Build history of the part. All positions in model axes, mm. A direction names the side the tool comes from. Coordinates: 2 decimals unless noted, no trailing zeros. Loops run counter-clockwise (first coordinate to the right, second up) from the corner with the lowest first, then second, coordinate; pieces in that order, holes last.
(1) Wall check: L1, parallel to Y at x = 0, z = 1.5; L2, parallel to Y at x = 0, z = -1. Give the ranges that are in metal, low to high.
(2) Flat gauge pins, fed straight in: P1, Ø10, axis at x = -23, z = 10, coming from the +Y side; P2, Ø18.5, axis at y = 19.5, z = 55, coming from the -X side; P3, Ø10, axis at x = 9, y = -2.5, coming from the -Z side; P4, Ø2, axis at y = 6.5, z = 42, coming from the -X side. Where does each tip first touch, or does it go through?
(3) Tool access for faces 4 (the face through (-20, -0.75, 45)), 5 (the face through (-7.14, -7, 72.57)), 6 (the face through (-9.213, -9.407, 64.333)), 7 (the face through (0.75, 20, 45)): list every direction of +Z, -Z, +X, -X, +Y, -Y with a clear straight run to the whole face (end or side of a thin tool).
(4) Slice it at A-A (z = 44). Give the cut face in (x, y), and give its area (3 significant figures).
(5) Two-plate mould, pull along Y, no slides. Class faces 1 (the face through (-8, -8, -5)), 2 (the face through (19.115, -18.713, 76.37)), 3 (the face through (-9.407, 9.213, 64.333)): pulls with the +Y half, pulls with the -Y half, needs draft (parallel to the pull), parting line crosses it, or undercut.
from build123d import *

# Parameters (mm, degrees)
AXLE_BASE_SKETCH_R        = 26
AXLE_DEPTH                = 77.5
GUARD_BASE_R              = 37.5
GUARD_DEPTH               = 5
INNER_AXLE_HOLE_BASE_R    = 10
INNER_AXLE_HOLE_DEPTH     = 83.5
BEND_START                = -64.5
BEND_ROOM_BASE_W          = 1.5
BEND_ROOM_BASE_H          = 75
BEND_ROOM_1_DEPTH         = 64.5
BEND_ROOM_2_COUNT         = 2
BEND_ROOM_2_ANGLE         = 90
EASY_REMOVAL_CHAMFER_SIZE = 4


with BuildPart() as part:
    # Axle base sketch → Axle (new body)
    with BuildSketch(Plane.XY):
        Circle(AXLE_BASE_SKETCH_R)
    extrude(amount=AXLE_DEPTH)

    # Guard base → Guard (add)
    with BuildSketch(Plane(origin=(0, 0, 0), x_dir=(-1, 0, 0), z_dir=(0, 0, -1))):
        Circle(GUARD_BASE_R)
    extrude(amount=GUARD_DEPTH)

    # Inner axle hole base → Inner axle hole (cut, through all)
    with BuildSketch(Plane.XY.offset(77.5)):
        Circle(INNER_AXLE_HOLE_BASE_R)
    extrude(amount=-INNER_AXLE_HOLE_DEPTH, mode=Mode.SUBTRACT)

    # Mate ring base → Mate rings (revolve)
    with BuildSketch(Plane(origin=(0, 0, 0), x_dir=(1, 0, 0), z_dir=(0, 1, 0))):
        Polygon((26, -77.5), (26.75, -76.75), (26.75, -76), (26, -75.25), align=None)
        Polygon((26, -71.75), (26.75, -71), (26.75, -70.25), (26, -69.5), align=None)
    revolve(axis=Axis((0, 0, 0), (0, 0, -1)))

    # Inner mass remove base → Inner mass remove (revolve, cut)
    with BuildSketch(Plane(origin=(0, 0, 0), x_dir=(0, 0, -1), z_dir=(1, 0, 0))):
        Polygon((-77.5, 0), (-59.5, -18), (-13, -18), (5, 0), align=None)
    revolve(axis=Axis((0, 0, 0), (0, 0, -1)), mode=Mode.SUBTRACT)

    # Bend room base → Bend room 1 (cut)
    with BuildSketch(Plane.XY.offset(77.5).offset(BEND_START)):
        Rectangle(BEND_ROOM_BASE_W, BEND_ROOM_BASE_H)
    bend_room_1 = extrude(amount=BEND_ROOM_1_DEPTH, mode=Mode.SUBTRACT)

    # Bend room 2: Bend room 1 ×2 about axis
    bend_room_2_axis = Axis((0, 0, 0), (0, 0, -1))
    for i in range(1, BEND_ROOM_2_COUNT):
        add(bend_room_1.rotate(bend_room_2_axis, i * BEND_ROOM_2_ANGLE / (BEND_ROOM_2_COUNT - 1)), mode=Mode.SUBTRACT)

    # Easy removal chamfer
    easy_removal_chamfer_edges = [part.edges().sort_by_distance(p)[0] for p in [
        (37.5, 0, 0),
    ]]
    chamfer(easy_removal_chamfer_edges, length=EASY_REMOVAL_CHAMFER_SIZE)


solid = part.part
Response values:
1. L1: y = -26 to -10, 10 to 26
1. L2: y = -34.5 to -10, 10 to 34.5
2. P1: stops at y = 18.76
2. P2: stops at x = -23.89
2. P3: stops at z = -5
2. P4: stops at x = -25.41
3. face 4: +Z, +X, -X
3. face 5: +Z, -Z
3. face 6: none
3. face 7: +Z, +Y, -Y
4. outline: (-25.99, -0.75) arc R26 ccw to (-0.75, -25.99) - (-0.75, -17.98) arc R18 cw to (-17.98, -0.75) - close; (-25.99, 0.75) - (-17.98, 0.75) arc R18 cw to (-0.75, 17.98) - (-0.75, 25.99) arc R26 ccw to start; (0.75, -25.99) arc R26 ccw to (25.99, -0.75) - (17.98, -0.75) arc R18 cw to (0.75, -17.98) - close; (0.75, 17.98) arc R18 cw to (17.98, 0.75) - (25.99, 0.75) arc R26 ccw to (0.75, 25.99) - close
4. area: 1,060 mm2
5. face 1: needs draft
5. face 2: pulls with the -Y half
5. face 3: undercut
